```python
from build123d import *

# Parameters (mm, degrees)
F1_DEPTH = 4
F3_R     = 5


with BuildPart() as f1:
    # F0 (on Top) → F1 (new body)
    with BuildSketch(Plane.XY):
        with BuildLine():
            ThreePointArc((-5.2846358413, 41.6185706289), (-4.227869293, 42.6976072612), (-2.9562644856, 43.5125286104))
            Line((-2.9562644856, 43.5125286104), (-17.160939287, 62.1069535454))
            ThreePointArc((-17.160939287, 62.1069535454), (-18.3698486288, 61.2181083005), (-19.5328025761, 60.2699280527))
            Line((-19.5328025761, 60.2699280527), (-5.2846358413, 41.6185706289))
        make_face()
        with BuildLine():
            ThreePointArc((-19.5328025761, 60.2699280527), (-18.3698486288, 61.2181083005), (-17.160939287, 62.1069535454))
            ThreePointArc((-17.160939287, 62.1069535454), (-8.9942035122, 66.1199983086), (0, 67.5))
            Line((0, 67.5), (0, 70.5))
            ThreePointArc((0, 70.5), (-32.9194358863, 39.8045044859), (-4.5977568287, 4.8218630864))
            Line((-4.5977568287, 4.8218630864), (0, 4.8218630864))
            Line((0, 4.8218630864), (0, 7.5))
            ThreePointArc((0, 7.5), (-8.9942035122, 8.8800016914), (-17.160939287, 12.8930464546))
            ThreePointArc((-17.160939287, 12.8930464546), (-18.3698486288, 13.7818916995), (-19.5328025761, 14.7300719473))
            ThreePointArc((-19.5328025761, 14.7300719473), (-30, 37.5), (-19.5328025761, 60.2699280527))
        make_face()
        with BuildLine():
            Line((-17.160939287, 12.8930464546), (-2.9562644856, 31.4874713896))
            ThreePointArc((-2.9562644856, 31.4874713896), (-4.227869293, 32.3023927388), (-5.2846358413, 33.3814293711))
            Line((-5.2846358413, 33.3814293711), (-19.5328025761, 14.7300719473))
            ThreePointArc((-19.5328025761, 14.7300719473), (-18.3698486288, 13.7818916995), (-17.160939287, 12.8930464546))
        make_face()
        with BuildLine():
            ThreePointArc((0, 4.5), (-2.3045044859, 4.5805641137), (-4.5977568287, 4.8218630864))
            Line((-4.5977568287, 4.8218630864), (-4.5977568287, 0))
            Line((-4.5977568287, 0), (0, 0))
            Line((0, 0), (0, 4.5))
        make_face()
        with BuildLine():
            Line((0, 4.5), (0, 4.8218630864))
            Line((0, 4.8218630864), (-4.5977568287, 4.8218630864))
            ThreePointArc((-4.5977568287, 4.8218630864), (-2.3045044859, 4.5805641137), (0, 4.5))
        make_face()
        with BuildLine():
            ThreePointArc((4.1952353927, 37.3), (-4.2, 37.5), (4.1952353927, 37.7))
            Line((4.1952353927, 37.7), (6.6970142601, 37.7))
            ThreePointArc((6.6970142601, 37.7), (3.4561068315, 43.2398018754), (-2.9562644856, 43.5125286104))
            ThreePointArc((-2.9562644856, 43.5125286104), (-4.227869293, 42.6976072612), (-5.2846358413, 41.6185706289))
            ThreePointArc((-5.2846358413, 41.6185706289), (-6.7, 37.5), (-5.2846358413, 33.3814293711))
            ThreePointArc((-5.2846358413, 33.3814293711), (-4.227869293, 32.3023927388), (-2.9562644856, 31.4874713896))
            ThreePointArc((-2.9562644856, 31.4874713896), (3.4561068315, 31.7601981246), (6.6970142601, 37.3))
            Line((6.6970142601, 37.3), (4.1952353927, 37.3))
        make_face()
    extrude(amount=F1_DEPTH)

    # F2: F1 across plane


with BuildPart() as f1_1:
    add(f1.part)
    add(f1.part.mirror(Plane.XZ))

    # F3
    f3_edges = [f1_1.edges().sort_by_distance(p)[0] for p in [
        (0, 7.5, 2),
        (-4.597757, -4.821863, 2),
        (-4.597757, 4.821863, 2),
        (0, -7.5, 2),
    ]]
    fillet(f3_edges, radius=F3_R)


solid = f1_1.part
```
Geometry check sheet. Reference: the model listing, model coordinates, mm. A direction names the side the tool comes from. Round coordinates to 2 decimals unless told otherwise and drop trailing zeros. Order: outer loops, then holes, each group sorted by start corner. A loop starts at its lowest first (then second) coordinate and runs counter-clockwise, first axis right, second up. Notation, with made-up numbers: (4, 40) -> (47, 40) arc R19 ccw to (47, 67) -> close; hole circle Ø7 at (47.25, -9). An arc over 180 degrees is marked (long way). Return JSON: item names as keys, results as strings. Group by question number.
Q1. Tool access check on faces 1 (the cylindrical face through (-6.7, -37.6, 2)), 2 (the cylindrical face through (-32.64, -42.36, 1.97)), 3 (the cylindrical face through (-1.188, 6.094, 2.028)). Record the directions out of +Z, -Z, +X, -X, +Y, -Y that give a thin tool (end or side, any length) a straight path to the whole face; none if there is none.
Q2. Section check A-A, the plane y = -39.5. Record the boundary of the cut face in (x, z), plus the area to 3 significant figures.
Q3. Release check for a two-part mould opening along Y. For faces 4 (the flat face through (-9.96, -52.68, 1.97)), 5 (the flat face through (-7, -6, 4)), 6 (the cylindrical face through (-10.93, 9.56, 1.97)) record: released by +Y, released by -Y, zero draft, split by the parting line, or undercut.
Q4. Section check C-C, the plane z = 1. Count the separate pieces of the cut face and the enclosed holes in it, plus the area to 3 significant figures.
Q5. Material ranges on probe 1 along X at (y, z) = (-37.5, 3.05); probe 2 along Y at (x, z) = (-21.5, 1.05); probe 3 along X at (y, z) = (-34, 1.7), recorded low to high. Write a range as from..to.
Q6. Section check D-D, the plane y = 11. Record the boundary of the cut face in (x, z).
Q7. Gauge pin test, flat ends, axial feed: pin 1 (1.3 mm diameter, centred on x = 5.5, z = 3, fed in from +Y); pin 2 (1 mm diameter, centred on x = -23.5, z = 1, fed in from +Y); pin 3 (1.3 mm diameter, centred on x = 5, z = 2.5, fed in from -Y). Record the tip position at first contact, or that the pin passes through.
Q8. Section check B-B, the plane x = -28. Record the boundary of the cut face in (y, z).
Numbers:
{
 "1": {"face 1": "+Z, -Z", "face 2": "+Z, -Z, -X", "face 3": "+Z, -Z, +X"},
 "2": {"outline": "(-32.94, 0) -> (-29.93, 0) -> (-29.93, 4) -> (-32.94, 4) -> close; (-6.39, 0) -> (-3.69, 0) -> (-3.69, 4) -> (-6.39, 4) -> close; (3.69, 0) -> (6.39, 0) -> (6.39, 4) -> (3.69, 4) -> close", "area": "33.6 mm^2"},
 "3": {"face 4": "undercut", "face 5": "zero draft", "face 6": "undercut"},
 "4": {"separate pieces": "1", "enclosed holes": "2", "area": "1,080 mm^2"},
 "5": {"probe 1": "-33..-30, -6.7..-4.2", "probe 2": "-62.53..-58.42, -16.58..-12.47, 12.47..16.58, 58.42..62.53", "probe 3": "-32.81..-29.8, -5.71..-2.32, 2.32..5.71"},
 "6": {"outline": "(-19.67, 0) -> (-14.06, 0) -> (-14.06, 4) -> (-19.67, 4) -> close"},
 "7": {"pin 1": "y = 42.12", "pin 2": "y = 61.16", "pin 3": "y = -42.6"},
 "8": {"outline": "(-54.96, 0) -> (-48.27, 0) -> (-48.27, 4) -> (-54.96, 4) -> close; (-26.73, 0) -> (-20.04, 0) -> (-20.04, 4) -> (-26.73, 4) -> close; (20.04, 0) -> (26.73, 0) -> (26.73, 4) -> (20.04, 4) -> close; (48.27, 0) -> (54.96, 0) -> (54.96, 4) -> (48.27, 4) -> close"}
}
